from build123d import *

# Parameters (mm, degrees)
F1_DEPTH = 4.6
F2_R     = 2


with BuildPart() as f1:
    # F0 (on Front) → F1 (new body, symmetric)
    with BuildSketch(Plane.XZ):
        Polygon((-43.125954, -18.449846), (-43.125954, -23.699846), (-33.125954, -23.699846), (-33.125954, -18.449846), (-34.519099, -18.449846), (-35.297526, -19.228273), (-38.125954, -22.0567), (-40.954381, -19.228273), (-41.732808, -18.449846), align=None)
    extrude(amount=F1_DEPTH, both=True)

    # F2
    f2_edges = [f1.edges().sort_by_distance(p)[0] for p in [
        (-38.125954, 0, -22.0567),
    ]]
    fillet(f2_edges, radius=F2_R)


solid = f1.part
Check sheet for the modelled part. Datum: model origin and axes. Units: mm. Round coordinates to 2 decimals unless told otherwise and drop trailing zeros. Order: outer loops, then holes, each group sorted by start corner. A loop starts at its lowest first (then second) coordinate and runs counter-clockwise, first axis right, second up. Notation, with made-up numbers: M 51.5,31.25 L 106.5,31.25 A25 cw 106.5,65.25 Z; hole C 75.5,85.25 d4. An arc over 180 degrees is marked long. One line per item, written item: value. Start each with the question number.
1. Gauge pin test, flat end, axial feed: P1, Ø1, axis at x = -36.5, y = 0.5, coming from the +Z side. Record the tip position at first contact, or that the pin passes through.
2. Section check A-A on z = -20.5. Enter the section's corners in (x, y), and give its area (3 significant figures).
3. Section check C-C on z = -19.6. Enter the section's corners in (x, y), and give its area (3 significant figures).
4. Section check D-D on x = -39. Enter the section's corners in (y, z), and give its area (3 significant figures).
5. Scan lines: line 1 along X through (y, z) = (3.75, -20.9); line 2 along X through (y, z) = (1, -19.1); line 3 along Z through (x, y) = (-35, 4.25). Record each from-to range of solid material in increasing order.
6. Release check for a two-part mould opening along X. For faces 1 (the flat face through (-43.126, 0, -21)), 2 (the flat face through (-40.62, -0.06, -19.56)), 3 (the flat face through (-38, -4.6, -22)), 4 (the cylindrical face through (-38.15, 0.06, -21.23)) record: released by +X, released by -X, zero draft, split by the parting line, or undercut.
7. Section check B-B on y = 0.5. Enter the section's corners in (x, z), and give its area (3 significant figures).
Results found:
1. P1: z = -19.93
2. outline: M -43.13,-4.6 L -39.68,-4.6 L -39.68,4.6 L -43.13,4.6 Z; M -36.57,-4.6 L -33.13,-4.6 L -33.13,4.6 L -36.57,4.6 Z
2. area: 63.4 mm^2
3. outline: M -43.13,-4.6 L -40.58,-4.6 L -40.58,4.6 L -43.13,4.6 Z; M -35.67,-4.6 L -33.13,-4.6 L -33.13,4.6 L -35.67,4.6 Z
3. area: 46.8 mm^2
4. outline: M -4.6,-23.7 L 4.6,-23.7 L 4.6,-21.03 L -4.6,-21.03 Z
4. area: 24.6 mm^2
5. line 1: -43.13 to -39.22, -37.03 to -33.13
5. line 2: -43.13 to -41.08, -35.17 to -33.13
5. line 3: -23.7 to -18.93
6. face 1: released by -X
6. face 2: undercut
6. face 3: zero draft
6. face 4: undercut
7. outline: M -43.13,-23.7 L -33.13,-23.7 L -33.13,-18.45 L -34.52,-18.45 L -35.3,-19.23 L -36.71,-20.64 A2 cw -39.54,-20.64 L -41.73,-18.45 L -43.13,-18.45 Z
7. area: 40.3 mm^2
